from build123d import *

# Parameters (mm, degrees)
SKETCH2_R          = 3.0734
CUT_EXTRUDE1_DEPTH = 15.494
SKETCH3_R          = 1.5494
CUT_EXTRUDE2_DEPTH = 17.3576
CHAMFER1_SIZE      = 3.81


with BuildPart() as part:
    # Sketch1 → Revolve1 (revolve)
    with BuildSketch(Plane.XY):
        Polygon((0, 0), (6.1214, 0), (6.1214, 9.8298), (9.4234, 9.8298), (9.4234, 11.8618), (7.1374, 11.8618), (7.1374, 14.3256), (9.4234, 14.3256), (9.4234, 16.3576), (0, 16.3576), (0, 9.8298), align=None)
    revolve(axis=Axis((0, 16.3576, 0), (0, -1, 0)))

    # Sketch2 → Cut-Extrude1 (cut)
    with BuildSketch(Plane(origin=(0, 16.3576, 0), x_dir=(1, 0, 0), z_dir=(0, 1, 0))):
        Circle(SKETCH2_R)
    extrude(amount=-CUT_EXTRUDE1_DEPTH, mode=Mode.SUBTRACT)

    # Sketch3 → Cut-Extrude2 (cut, through all)
    with BuildSketch(Plane.XZ):
        Circle(SKETCH3_R)
    extrude(amount=-CUT_EXTRUDE2_DEPTH, mode=Mode.SUBTRACT)

    # Chamfer1
    chamfer1_edges = [part.edges().sort_by_distance(p)[0] for p in [
        (-3.0734, 16.3576, 0),
    ]]
    chamfer(chamfer1_edges, length=CHAMFER1_SIZE)


solid = part.part
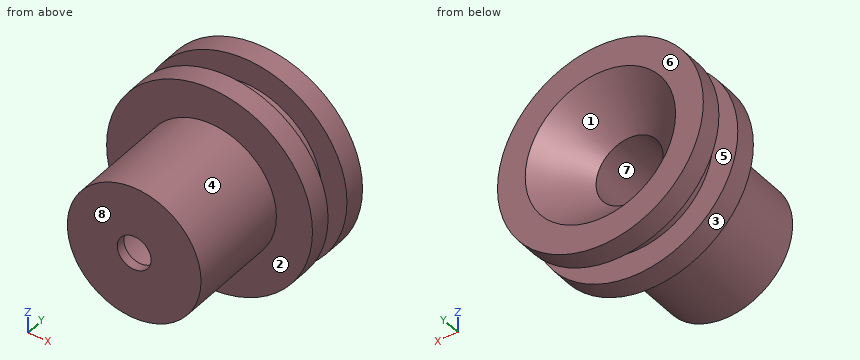
For this review, take the finished solid that the model builds, in its own axes (mm). Face numbers are marked on the shaded views. A direction names the side the tool comes from. Round coordinates to 2 decimals unless told otherwise and drop trailing zeros. Write each loop counter-clockwise with the first axis right and the second up, starting at its lowest first coordinate (ties: lowest second). Pieces come first, ordered by that corner, then holes. Notation, with made-up numbers: (-35.5, 27) - (-25.5, 27) arc R18 ccw to (-25.5, 33) - close; hole circle Ø6 at (24.25, -38.5). An arc over 180 degrees is marked (long way). Use a Markdown table: item, result.
Q1. Machinability: for the marked faces 4, 5, 6, 7 and 8, which of the approach directions +Z, -Z, +X, -X, +Y, -Y give a long, thin tool a straight path to every point of the face, cutting with its end or side? Answer none if there is none.
Derived:
| item | result |
|---|---|
| face 4 | -Y |
| face 5 | none |
| face 6 | +Z, -Z, +X, -X, +Y |
| face 7 | +Y |
| face 8 | +Z, -Z, +X, -X, -Y |
Q2. We need section A-A (z = 0). Give the boundary of the cut face in (x, y), plus the area to 3 significant figures.
Derived:
| item | result |
|---|---|
| outline | (-9.42, 9.83) - (-6.12, 9.83) - (-6.12, 0) - (-1.55, 0) - (-1.55, 0.86) - (-3.07, 0.86) - (-3.07, 12.55) - (-6.88, 16.36) - (-9.42, 16.36) - (-9.42, 14.33) - (-7.14, 14.33) - (-7.14, 11.86) - (-9.42, 11.86) - close; (1.55, 0) - (6.12, 0) - (6.12, 9.83) - (9.42, 9.83) - (9.42, 11.86) - (7.14, 11.86) - (7.14, 14.33) - (9.42, 14.33) - (9.42, 16.36) - (6.88, 16.36) - (3.07, 12.55) - (3.07, 0.86) - (1.55, 0.86) - close |
| area | 120 mm2 |
Q3. Clearance check with flat-ended pins moving along their axes: pin 1 (2 mm diameter, centred on x = -6, y = 7.5, fed in from +Z); pin 2 (4 mm diameter, centred on x = 5, y = 12.5, fed in from -Z); pin 3 (6 mm diameter, centred on y = 2, z = -6, fed in from +X). State where each tip first meets the part, or that it passes through.
Derived:
| item | result |
|---|---|
| pin 1 | stops at z = 3.53 |
| pin 2 | stops at z = -8.9 |
| pin 3 | stops at x = 5.34 |
Q4. We need section D-D (y = 13.5). Give the boundary of the cut face in (x, z), plus the area to 3 significant figures.
Derived:
| item | result |
|---|---|
| outline | circle Ø14.27 at (0, 0); hole circle Ø8.05 at (0, 0) |
| area | 109 mm2 |
Q5. The part is to be moulded in two halves that separate along X. For the marked faces 1, 2 and 3, say which applies: pulls with the +X half, pulls with the -X half, needs draft (parallel to the pull), parting line crosses it, or undercut.
Derived:
| item | result |
|---|---|
| face 1 | undercut |
| face 2 | needs draft |
| face 3 | parting line crosses it |
Q6. Wall thickness on line 1 along Z through (x, y) = (0, 4.5); line 2 along Y through (x, z) = (-6, 4); line 3 along Z through (x, y) = (0, 0.65): over which ranges is each line inside the solid? List them lowest first.
Derived:
| item | result |
|---|---|
| line 1 | z = -6.12 to -3.07, 3.07 to 6.12 |
| line 2 | y = 9.83 to 11.86, 14.33 to 16.36 |
| line 3 | z = -6.12 to -1.55, 1.55 to 6.12 |
Q7. We need section C-C (y = 8.25). Give the boundary of the cut face in (x, z), plus the area to 3 significant figures.
Derived:
| item | result |
|---|---|
| outline | circle Ø12.24 at (0, 0); hole circle Ø6.15 at (0, 0) |
| area | 88.0 mm2 |
Q8. We need section B-B (x = 0). Give the boundary of the cut face in (y, z).
Derived:
| item | result |
|---|---|
| outline | (0, -6.12) - (9.83, -6.12) - (9.83, -9.42) - (11.86, -9.42) - (11.86, -7.14) - (14.33, -7.14) - (14.33, -9.42) - (16.36, -9.42) - (16.36, -6.88) - (12.55, -3.07) - (0.86, -3.07) - (0.86, -1.55) - (0, -1.55) - close; (0, 1.55) - (0.86, 1.55) - (0.86, 3.07) - (12.55, 3.07) - (16.36, 6.88) - (16.36, 9.42) - (14.33, 9.42) - (14.33, 7.14) - (11.86, 7.14) - (11.86, 9.42) - (9.83, 9.42) - (9.83, 6.12) - (0, 6.12) - close |
